```python
from build123d import *

# Parameters (mm, degrees)
SKETCH2_R           = 1.65
SKETCH2_R_2         = 11
SKETCH2_R_3         = 3
SKETCH2_R_4         = 2.25
SKETCH2_R_5         = 2
BOSS_EXTRUDE1_DEPTH = 3.8


with BuildPart() as part:
    # Sketch2 → Boss-Extrude1 (new body)
    with BuildSketch(Plane.XY):
        with BuildLine():
            Line((165, 115), (165, 60))
            Line((165, 60), (158, 60))
            Line((158, 60), (158, -60))
            Line((158, -60), (165, -60))
            Line((165, -60), (165, -117.5))
            ThreePointArc((165, -117.5), (156.213203436, -138.713203436), (135, -147.5))
            Line((135, -147.5), (-135, -147.5))
            ThreePointArc((-135, -147.5), (-156.213203436, -138.713203436), (-165, -117.5))
            Line((-165, -117.5), (-165, -60))
            Line((-165, -60), (-158, -60))
            Line((-158, -60), (-158, 60))
            Line((-158, 60), (-165, 60))
            Line((-165, 60), (-165, 115))
            ThreePointArc((-165, 115), (-156.213203436, 136.213203436), (-135, 145))
            Line((-135, 145), (-71.563974327, 145))
            Line((-71.563974327, 145), (-25.002785582, 94.922799803))
            Line((-25.002785582, 94.922799803), (25.002785582, 94.922799803))
            Line((25.002785582, 94.922799803), (71.563974327, 145))
            Line((71.563974327, 145), (135, 145))
            ThreePointArc((135, 145), (156.213203436, 136.213203436), (165, 115))
        make_face()
        with Locations(Location((-129.334802826, 110, 0), (0, 0, 180))):
            Circle(SKETCH2_R, mode=Mode.SUBTRACT)
        with Locations(Location((-100.665197174, 110, 0), (0, 0, 180))):
            Circle(SKETCH2_R, mode=Mode.SUBTRACT)
        with Locations(Location((129.334802826, 110, 0), (0, 0, 180))):
            Circle(SKETCH2_R, mode=Mode.SUBTRACT)
        with Locations(Location((100.665197174, 110, 0), (0, 0, 180))):
            Circle(SKETCH2_R, mode=Mode.SUBTRACT)
        with Locations(Location((129.334802826, -110, 0), (0, 0, 180))):
            Circle(SKETCH2_R, mode=Mode.SUBTRACT)
        with Locations(Location((100.665197174, -110, 0), (0, 0, 180))):
            Circle(SKETCH2_R, mode=Mode.SUBTRACT)
        with Locations(Location((-129.334802826, -110, 0), (0, 0, 180))):
            Circle(SKETCH2_R, mode=Mode.SUBTRACT)
        with Locations(Location((-100.665197174, -110, 0), (0, 0, 180))):
            Circle(SKETCH2_R, mode=Mode.SUBTRACT)
        with Locations(Location((115, 110, 0), (0, 0, 180))):
            Circle(SKETCH2_R_2, mode=Mode.SUBTRACT)
        with Locations(Location((-115, 110, 0), (0, 0, 180))):
            Circle(SKETCH2_R_2, mode=Mode.SUBTRACT)
        with Locations(Location((115, -110, 0), (0, 0, 180))):
            Circle(SKETCH2_R_2, mode=Mode.SUBTRACT)
        with Locations(Location((-115, -110, 0), (0, 0, 180))):
            Circle(SKETCH2_R_2, mode=Mode.SUBTRACT)
        with Locations(Location((-105, 80, 0), (0, 0, 180))):
            Circle(SKETCH2_R_3, mode=Mode.SUBTRACT)
        with Locations(Location((105, 80, 0), (0, 0, 180))):
            Circle(SKETCH2_R_3, mode=Mode.SUBTRACT)
        with Locations(Location((105, -80, 0), (0, 0, 180))):
            Circle(SKETCH2_R_3, mode=Mode.SUBTRACT)
        with Locations(Location((-105, -80, 0), (0, 0, 180))):
            Circle(SKETCH2_R_3, mode=Mode.SUBTRACT)
        with Locations(Location((150.121259344, -25.5, 0), (0, 0, 180))):
            Circle(SKETCH2_R, mode=Mode.SUBTRACT)
        with Locations(Location((150.121259344, 25.5, 0), (0, 0, 180))):
            Circle(SKETCH2_R, mode=Mode.SUBTRACT)
        with Locations(Location((-150.121259344, -25.5, 0), (0, 0, 180))):
            Circle(SKETCH2_R, mode=Mode.SUBTRACT)
        with Locations(Location((-150.121259344, 25.5, 0), (0, 0, 180))):
            Circle(SKETCH2_R, mode=Mode.SUBTRACT)
        with Locations(Location((-55.73, -14.995, 0), (0, 0, 180))):
            Circle(SKETCH2_R_4, mode=Mode.SUBTRACT)
        with Locations(Location((-55.73, 14.895, 0), (0, 0, 180))):
            Circle(SKETCH2_R_4, mode=Mode.SUBTRACT)
        with Locations(Location((-79.79, 14.895, 0), (0, 0, 180))):
            Circle(SKETCH2_R_4, mode=Mode.SUBTRACT)
        with Locations(Location((-79.79, -14.995, 0), (0, 0, 180))):
            Circle(SKETCH2_R_4, mode=Mode.SUBTRACT)
        with Locations(Location((79.79, -14.995, 0), (0, 0, 180))):
            Circle(SKETCH2_R_4, mode=Mode.SUBTRACT)
        with Locations(Location((55.73, -14.995, 0), (0, 0, 180))):
            Circle(SKETCH2_R_4, mode=Mode.SUBTRACT)
        with Locations(Location((55.73, 14.895, 0), (0, 0, 180))):
            Circle(SKETCH2_R_4, mode=Mode.SUBTRACT)
        with Locations(Location((79.79, 14.895, 0), (0, 0, 180))):
            Circle(SKETCH2_R_4, mode=Mode.SUBTRACT)
        with Locations(Location((56, 120, 0), (0, 0, 180))):
            Circle(SKETCH2_R_4, mode=Mode.SUBTRACT)
        with Locations(Location((0, 88.922799803, 0), (0, 0, 180))):
            Circle(SKETCH2_R_5, mode=Mode.SUBTRACT)
        with Locations(Location((-56, 120, 0), (0, 0, 180))):
            Circle(SKETCH2_R_4, mode=Mode.SUBTRACT)
        with Locations(Location((155.24999999, 66.777335257, 0), (0, 0, 180))):
            Circle(SKETCH2_R_4, mode=Mode.SUBTRACT)
        with Locations(Location((155.24999999, 89.256565873, 0), (0, 0, 180))):
            Circle(SKETCH2_R_4, mode=Mode.SUBTRACT)
        with Locations(Location((155.24999999, -66.572399887, 0), (0, 0, 180))):
            Circle(SKETCH2_R_4, mode=Mode.SUBTRACT)
        with Locations(Location((155.24999999, -89.051630503, 0), (0, 0, 180))):
            Circle(SKETCH2_R_4, mode=Mode.SUBTRACT)
        with Locations(Location((104.427600113, -138.94999999, 0), (0, 0, 180))):
            Circle(SKETCH2_R_4, mode=Mode.SUBTRACT)
        with Locations(Location((81.948369497, -138.94999999, 0), (0, 0, 180))):
            Circle(SKETCH2_R_4, mode=Mode.SUBTRACT)
        with Locations(Location((-131.400317146, -128.880285492, 0), (0, 0, 180))):
            Circle(SKETCH2_R_4, mode=Mode.SUBTRACT)
        with Locations(Location((-150.638323589, -107.961051525, 0), (0, 0, 180))):
            Circle(SKETCH2_R_4, mode=Mode.SUBTRACT)
        with Locations(Location((-150.638323589, 105.461051525, 0), (0, 0, 180))):
            Circle(SKETCH2_R_5, mode=Mode.SUBTRACT)
        with Locations(Location((-131.400317146, 126.380285492, 0), (0, 0, 180))):
            Circle(SKETCH2_R_5, mode=Mode.SUBTRACT)
        with Locations(Location((-73.437500654, 136.44999999, 0), (0, 0, 180))):
            Circle(SKETCH2_R_4, mode=Mode.SUBTRACT)
        with Locations(Location((-95.91673127, 136.44999999, 0), (0, 0, 180))):
            Circle(SKETCH2_R_4, mode=Mode.SUBTRACT)
        with Locations(Location((95.99157444, 136.44999999, 0), (0, 0, 180))):
            Circle(SKETCH2_R_4, mode=Mode.SUBTRACT)
        with Locations(Location((73.512343824, 136.44999999, 0), (0, 0, 180))):
            Circle(SKETCH2_R_4, mode=Mode.SUBTRACT)
        with BuildLine():
            Line((113.717640114, -47.179866734), (93.717640114, -47.179866734))
            ThreePointArc((93.717640114, -47.179866734), (89.474999427, -45.422507421), (87.717640114, -41.179866734))
            Line((87.717640114, -41.179866734), (87.717640114, 41.179866734))
            ThreePointArc((87.717640114, 41.179866734), (89.474999427, 45.422507421), (93.717640114, 47.179866734))
            Line((93.717640114, 47.179866734), (113.717640114, 47.179866734))
            ThreePointArc((113.717640114, 47.179866734), (117.960280801, 45.422507421), (119.717640114, 41.179866734))
            Line((119.717640114, 41.179866734), (119.717640114, -41.179866734))
            ThreePointArc((119.717640114, -41.179866734), (117.960280801, -45.422507421), (113.717640114, -47.179866734))
        make_face(mode=Mode.SUBTRACT)
        with BuildLine():
            Line((-113.717640114, 47.179866734), (-93.717640114, 47.179866734))
            ThreePointArc((-93.717640114, 47.179866734), (-89.474999427, 45.422507421), (-87.717640114, 41.179866734))
            Line((-87.717640114, 41.179866734), (-87.717640114, -41.179866734))
            ThreePointArc((-87.717640114, -41.179866734), (-89.474999427, -45.422507421), (-93.717640114, -47.179866734))
            Line((-93.717640114, -47.179866734), (-113.717640114, -47.179866734))
            ThreePointArc((-113.717640114, -47.179866734), (-117.960280801, -45.422507421), (-119.717640114, -41.179866734))
            Line((-119.717640114, -41.179866734), (-119.717640114, 41.179866734))
            ThreePointArc((-119.717640114, 41.179866734), (-117.960280801, 45.422507421), (-113.717640114, 47.179866734))
        make_face(mode=Mode.SUBTRACT)
    extrude(amount=BOSS_EXTRUDE1_DEPTH)


solid = part.part
```
Geometry check sheet. Reference: the model listing, model coordinates, mm. A direction names the side the tool comes from. Coordinates: 2 decimals unless noted, no trailing zeros. Order: outer loops, then holes, each group sorted by start corner. A loop starts at its lowest first (then second) coordinate and runs counter-clockwise, first axis right, second up. Notation, with made-up numbers: (36.5, 24) - (48.5, 24) arc R30 cw to (48.5, 59) - close; hole circle Ø5 at (12, 4). An arc over 180 degrees is marked (long way). Answer as a JSON object with one key per item and string values. Group by question number.
Item 1: Scan lines: probe 1 along X at (y, z) = (-25.5, 2.8); probe 2 along X at (y, z) = (-80, 3.05); probe 3 along X at (y, z) = (20, 3.2). Record each from-to range of solid material in increasing order.
Item 2: Tool access check on faces 4 (the face through (126, -110, 2)), 5 (the face through (-48.6, 120.3, 1.9)). Record the directions out of +Z, -Z, +X, -X, +Y, -Y that give a thin tool (end or side, any length) a straight path to the whole face; none if there is none.
Item 3: Sectioned sample at B-B, the plane x = 6. Record the cut outline in (y, z).
Item 4: Sectioned sample at C-C, the plane z = 1.6. Give the number of separate pieces and of enclosed holes in the cut face, and give its area (3 significant figures).
Item 5: Depth check by flat-ended pin: pin 1 Ø6 at (x, y) = (155.25, -66.57) entering from -Z. Enter the tip coordinate at first touch or a pass-through.
Item 6: Sectioned sample at D-D, the plane x = -45. Record the cut outline in (y, z).
Item 7: Sectioned sample at A-A, the plane y = 34. Record the cut outline in (x, z), and give its area (3 significant figures).
Item 8: Draft check along Y on faces 1 (the face through (-104, 110, 2)), 2 (the face through (155.979, 136.445, 1.873)), 3 (the face through (-155.979, -138.945, 1.873)). Enter one of: +Y half, -Y half, draft (parallel to the pull), parting line (faces both ways), or undercut.
Resolved:
{
 "1": {"probe 1": "-158 to -151.77, -148.47 to -119.72, -87.72 to 87.72, 119.72 to 148.47, 151.77 to 158", "probe 2": "-165 to -108, -102 to 102, 108 to 165", "probe 3": "-158 to -119.72, -87.72 to 87.72, 119.72 to 158"},
 "2": {"face 4": "+Z, -Z", "face 5": "+Z, -Z, +Y"},
 "3": {"outline": "(-147.5, 0) - (94.92, 0) - (94.92, 3.8) - (-147.5, 3.8) - close"},
 "4": {"separate pieces": "1", "enclosed holes": "47", "area": "81,100 mm^2"},
 "5": {"pin 1": "z = 0"},
 "6": {"outline": "(-147.5, 0) - (116.43, 0) - (116.43, 3.8) - (-147.5, 3.8) - close"},
 "7": {"outline": "(-158, 0) - (-119.72, 0) - (-119.72, 3.8) - (-158, 3.8) - close; (-87.72, 0) - (87.72, 0) - (87.72, 3.8) - (-87.72, 3.8) - close; (119.72, 0) - (158, 0) - (158, 3.8) - (119.72, 3.8) - close", "area": "958 mm^2"},
 "8": {"face 1": "undercut", "face 2": "+Y half", "face 3": "-Y half"}
}
